```python
from build123d import *
from build123d.topology import SkipClean

# Parameters (mm, degrees)
ESTRUSIONE_ESTRUSIONE1_DEPTH  = 6
ESTRUSIONE_ESTRUSIONE3_START  = -11
SCHIZZO3_R                    = 5
SCHIZZO3_R_2                  = 2.65
ESTRUSIONE_ESTRUSIONE3_DEPTH  = 11
SCHIZZO5_R                    = 0.925
ESTRUSIONE_ESTRUSIONE4_DEPTH  = 20
SCHIZZO12_W                   = 8
SCHIZZO12_H                   = 6
ESTRUSIONE_ESTRUSIONE6_DEPTH  = 2
SCHIZZO13_W                   = 6
SCHIZZO13_H                   = 2
ESTRUSIONE_ESTRUSIONE7_DEPTH  = 3
RACCORDO2_R                   = 2.5
SCHIZZO14_R                   = 1.75
SCHIZZO14_R_2                 = 0.925
TAGLIO_ESTRUSIONE7_DEPTH      = 25
SCHIZZO15_W                   = 6
SCHIZZO15_H                   = 8
ESTRUSIONE_ESTRUSIONE8_DEPTH  = 24
SCHIZZO16_W                   = 6
SCHIZZO16_H                   = 2
ESTRUSIONE_ESTRUSIONE9_DEPTH  = 7.999994
SCHIZZO17_R                   = 1.25
TAGLIO_ESTRUSIONE8_DEPTH      = 25
RACCORDO3_R                   = 10
RACCORDO4_R                   = 10
RACCORDO5_R                   = 10
RACCORDO6_R                   = 2.5
SCHIZZO18_R                   = 1.75
TAGLIO_ESTRUSIONE9_DEPTH      = 39.431359843
SCHIZZO20_W                   = 20
SCHIZZO20_H                   = 19.30891557
TAGLIO_ESTRUSIONE10_DEPTH     = 39.431359843
SCHIZZO21_W                   = 5
SCHIZZO21_H                   = 10
ESTRUSIONE_ESTRUSIONE10_DEPTH = 9.5
SCHIZZO22_W                   = 5
SCHIZZO22_H                   = 10
ESTRUSIONE_ESTRUSIONE11_DEPTH = 15
RACCORDO7_R                   = 5
RACCORDO8_R                   = 10
RACCORDO9_R                   = 5
ESTRUSIONE_ESTRUSIONE13_START = 5
SCHIZZO24_R                   = 5
SCHIZZO24_R_2                 = 2.6
ESTRUSIONE_ESTRUSIONE13_DEPTH = 5
SCHIZZO26_R                   = 1.75
TAGLIO_ESTRUSIONE12_DEPTH     = 39.29124471
RACCORDO10_R                  = 5


with BuildPart() as part:
    # Schizzo1 → Estrusione-Estrusione1 (new body)
    with BuildSketch(Plane.XY):
        with BuildLine():
            Line((0, 0), (-20, 0))
            Line((-20, 0), (-10, 10))
            Line((-10, 10), (10, 10))
            ThreePointArc((10, 10), (15, 5), (10, 0))
            Line((10, 0), (0, 0))
        make_face()
    extrude(amount=ESTRUSIONE_ESTRUSIONE1_DEPTH)

    # Schizzo3 → Estrusione-Estrusione3 (add)
    with SkipClean():  # the faces are left unmerged after this step: merging them gives an invalid solid
        with BuildSketch(Plane.XY.offset(6).offset(ESTRUSIONE_ESTRUSIONE3_START)):
            with Locations(Location((10, 5, 0), (0, 0, 270))):
                Circle(SCHIZZO3_R)
            with Locations((10, 5)):
                Circle(SCHIZZO3_R_2, mode=Mode.SUBTRACT)
        extrude(amount=ESTRUSIONE_ESTRUSIONE3_DEPTH)



with BuildPart() as body_2:
    # Schizzo5 → Estrusione-Estrusione4 (new body)
    with BuildSketch(Plane(origin=(0, 0, 0), x_dir=(-0.7071067811865476, 0.7071067811865476, 0), z_dir=(0.7071067811865476, 0.7071067811865476, 0))):
        with Locations((18.142135624, 3)):
            Circle(SCHIZZO5_R)
    extrude(amount=-ESTRUSIONE_ESTRUSIONE4_DEPTH)

    # Schizzo12 → Estrusione-Estrusione6 (add)
    with BuildSketch(Plane(origin=(0, 0, 0), x_dir=(-0.7071067811865476, 0.7071067811865476, 0), z_dir=(0.7071067811865476, 0.7071067811865476, 0))):
        with Locations((18.142135624, 3)):
            Rectangle(SCHIZZO12_W, SCHIZZO12_H)
    extrude(amount=ESTRUSIONE_ESTRUSIONE6_DEPTH)


with BuildPart() as part_1:
    with SkipClean():  # the faces are left unmerged after this step: merging them gives an invalid solid
        add(part.part)

        add(body_2.part)  # Estrusione-Estrusione7 merges body 2
        # Schizzo13 → Estrusione-Estrusione7 (add)
        with BuildSketch(Plane(origin=(-10, 10, 0), x_dir=(0, 0, -1), z_dir=(0.7071067811865477, -0.7071067811865475, 0))):
            with Locations((-3, 1)):
                Rectangle(SCHIZZO13_W, SCHIZZO13_H)
        extrude(amount=ESTRUSIONE_ESTRUSIONE7_DEPTH)

    # Raccordo2
    raccordo2_edges = [part_1.edges().sort_by_distance(p)[0] for p in [
        (-14.949747468, 16.363961031, 0),
        (-14.949747468, 16.363961031, 6),
    ]]
    fillet(raccordo2_edges, radius=RACCORDO2_R)

    # Schizzo14 → Taglio-Estrusione7 (cut)
    # profile 1 of 2: a face of its own
    with SkipClean():  # the faces are left unmerged after this step: merging them gives an invalid solid
        with BuildSketch(Plane(origin=(1.414213562, 1.414213562, 0), x_dir=(0, 0, -1), z_dir=(0.7071067811865476, 0.7071067811865476, 0))):
            with Locations(Location((-3, 18.142135624, 0), (0, 0, 90))):
                Circle(SCHIZZO14_R)
            with Locations((-3, 18.142135624)):
                Circle(SCHIZZO14_R_2, mode=Mode.SUBTRACT)
        # profile 2 of 2: a face of its own
        with BuildSketch(Plane(origin=(1.414213562, 1.414213562, 0), x_dir=(0, 0, -1), z_dir=(0.7071067811865476, 0.7071067811865476, 0))):
            with Locations((-3, 18.142135624)):
                Circle(SCHIZZO14_R_2)
        extrude(amount=-TAGLIO_ESTRUSIONE7_DEPTH, mode=Mode.SUBTRACT)

    # Schizzo15 → Estrusione-Estrusione8 (add)
    with SkipClean():  # the faces are left unmerged after this step: merging them gives an invalid solid
        with BuildSketch(Plane(origin=(0, 0, 0), x_dir=(0, 0, 1), z_dir=(-0.7071067811865477, -0.7071067811865475, 0))):
            with Locations((3, 10.142135624)):
                Rectangle(SCHIZZO15_W, SCHIZZO15_H)
        extrude(amount=ESTRUSIONE_ESTRUSIONE8_DEPTH)

    # Schizzo16 → Estrusione-Estrusione9 (add)
    with SkipClean():  # the faces are left unmerged after this step: merging them gives an invalid solid
        with BuildSketch(Plane(origin=(-10, 10, 0), x_dir=(0, 0, 1), z_dir=(-0.7071067811865477, 0.7071067811865475, 0))):
            with Locations((3, -23)):
                Rectangle(SCHIZZO16_W, SCHIZZO16_H)
        extrude(amount=ESTRUSIONE_ESTRUSIONE9_DEPTH)

    # Schizzo17 → Taglio-Estrusione8 (cut)
    with SkipClean():  # the faces are left unmerged after this step: merging them gives an invalid solid
        with BuildSketch(Plane(origin=(-16.970562748, -16.970562748, 0), x_dir=(0, 0, 1), z_dir=(-0.7071067811865477, -0.7071067811865474, 0))):
            with Locations(Location((3, 18.142135624, 0), (0, 0, 270))):
                Circle(SCHIZZO17_R)
        extrude(amount=-TAGLIO_ESTRUSIONE8_DEPTH, mode=Mode.SUBTRACT)

    # Raccordo3
    # the kernel refuses this fillet: 10 mm, written as the material it takes off along each edge
    with BuildSketch(Plane(origin=(-21.313708499, -12.627416998, -25), x_dir=(0.7071067811865475, 0.7071067811865475, 0), z_dir=(0, 0, 1))) as raccordo3_piece_1:
        with BuildLine():
            CenterArc((RACCORDO3_R, RACCORDO3_R), RACCORDO3_R, 180, 90)
            Line((0, RACCORDO3_R), (0, 0))
            Line((0, 0), (RACCORDO3_R, 0))
        make_face()
    extrude(amount=56, mode=Mode.SUBTRACT)

    # Raccordo4
    raccordo4_edges = [part_1.edges().sort_by_distance(p)[0] for p in [
        (-8.686291501, 0, 3),
    ]]
    fillet(raccordo4_edges, radius=RACCORDO4_R)

    # Raccordo5
    raccordo5_edges = [part_1.edges().sort_by_distance(p)[0] for p in [
        (-7.171572875, 10, 3),
    ]]
    fillet(raccordo5_edges, radius=RACCORDO5_R)

    # Raccordo6
    raccordo6_edges = [part_1.edges().sort_by_distance(p)[0] for p in [
        (-31.920305974, -0.60660596, 6),
        (-31.920305974, -0.60660596, 0),
    ]]
    fillet(raccordo6_edges, radius=RACCORDO6_R)

    # Schizzo18 → Taglio-Estrusione9 (cut, through all)
    with BuildSketch(Plane.XY.offset(6)):
        with Locations((10, 5)):
            Circle(SCHIZZO18_R)
    extrude(amount=-TAGLIO_ESTRUSIONE9_DEPTH, mode=Mode.SUBTRACT)

    # Schizzo20 → Taglio-Estrusione10 (cut, through all)
    with BuildSketch(Plane(origin=(0, 0, -5), x_dir=(-1, 0, 0), z_dir=(0, 0, -1))):
        with Locations((-10, 5)):
            Rectangle(SCHIZZO20_W, SCHIZZO20_H)
    extrude(amount=-TAGLIO_ESTRUSIONE10_DEPTH, mode=Mode.SUBTRACT)

    # Schizzo21 → Estrusione-Estrusione10 (add)
    with BuildSketch(Plane.XY.offset(6)):
        with Locations((-0.529437252, 5)):
            Rectangle(SCHIZZO21_W, SCHIZZO21_H)
    extrude(amount=ESTRUSIONE_ESTRUSIONE10_DEPTH)

    # Schizzo22 → Estrusione-Estrusione11 (add)
    with BuildSketch(Plane(origin=(1.970562748, 0, 0), x_dir=(0, 0, -1), z_dir=(1, 0, 0))):
        with Locations((-13, 5)):
            Rectangle(SCHIZZO22_W, SCHIZZO22_H)
    extrude(amount=ESTRUSIONE_ESTRUSIONE11_DEPTH)

    # Raccordo7
    # the kernel refuses this fillet: 5 mm, written as the material it takes off along each edge
    with BuildSketch(Plane(origin=(1.970562748, 19.944379675, 6), x_dir=(-1, 0, 0), z_dir=(0, -1, 0))) as raccordo7_piece_1:
        with BuildLine():
            CenterArc((5, -3.97775187), RACCORDO7_R, 127.292729202, 52.707270798)
            Line((0, -3.97775187), (-0.1, -3.97775187))
            Line((-0.1, -3.97775187), (-0.1, 0))
            Line((-0.1, 0), (0, 0.1))
            ThreePointArc((0, 0.1), (0.985281374, 0.1), (1.909974003, 0.079555037))
            Line((1.909974003, 0.079555037), (1.970562748, 0))
        make_face()
    extrude(amount=29.88875935, mode=Mode.SUBTRACT)
    with BuildSketch(Plane(origin=(16.970562748, 0, -2), x_dir=(0, 1, 0), z_dir=(0, 0, 1))) as raccordo7_piece_2:
        with BuildLine():
            CenterArc((RACCORDO7_R, RACCORDO7_R), RACCORDO7_R, 180, 90)
            Line((0, RACCORDO7_R), (-RACCORDO7_R * 0.02, RACCORDO7_R))
            Line((-RACCORDO7_R * 0.02, RACCORDO7_R), (-RACCORDO7_R * 0.02, -RACCORDO7_R * 0.02))
            Line((-RACCORDO7_R * 0.02, -RACCORDO7_R * 0.02), (RACCORDO7_R, -RACCORDO7_R * 0.02))
            Line((RACCORDO7_R, -RACCORDO7_R * 0.02), (RACCORDO7_R, 0))
        make_face()
    extrude(amount=30, mode=Mode.SUBTRACT)
    with BuildSketch(Plane(origin=(16.970562748, 10, 28), x_dir=(-1, 0, 0), z_dir=(0, 0, -1))) as raccordo7_piece_3:
        with BuildLine():
            CenterArc((RACCORDO7_R, -RACCORDO7_R), RACCORDO7_R, 90, 90)
            Line((0, -RACCORDO7_R), (-RACCORDO7_R * 0.02, -RACCORDO7_R))
            Line((-RACCORDO7_R * 0.02, -RACCORDO7_R), (-RACCORDO7_R * 0.02, RACCORDO7_R * 0.02))
            Line((-RACCORDO7_R * 0.02, RACCORDO7_R * 0.02), (RACCORDO7_R, RACCORDO7_R * 0.02))
            Line((RACCORDO7_R, RACCORDO7_R * 0.02), (RACCORDO7_R, 0))
        make_face()
    extrude(amount=30, mode=Mode.SUBTRACT)

    # Raccordo8
    # the kernel refuses this fillet: 10 mm, written as the material it takes off along each edge
    with BuildSketch(Plane(origin=(-3.029437252, -24.968730444, 15.5), x_dir=(1, 0, 0), z_dir=(0, 1, 0))) as raccordo8_piece_1:
        with BuildLine():
            CenterArc((9.987492178, 10), RACCORDO8_R, 182.865983983, 87.134016017)
            Line((0, 9.5), (-0.199749844, 9.49))
            ThreePointArc((-0.199749844, 9.49), (-0.2, 4.75), (-0.2, 0))
            Line((-0.2, 0), (0, -0.2))
            Line((0, -0.2), (9.987492178, -0.2))
            Line((9.987492178, -0.2), (9.987492178, 0))
        make_face()
    extrude(amount=59.937460889, mode=Mode.SUBTRACT)

    # Raccordo9
    raccordo9_edges = [part_1.edges().sort_by_distance(p)[0] for p in [
        (-3.029437252, 5, 6),
    ]]
    fillet(raccordo9_edges, radius=RACCORDO9_R)

    # Schizzo24 → Estrusione-Estrusione13 (add)
    with BuildSketch(Plane(origin=(0, 0, 10.5), x_dir=(-1, 0, 0), z_dir=(0, 0, -1)).offset(ESTRUSIONE_ESTRUSIONE13_START)):
        with Locations(Location((-11.970562748, 5, 0), (0, 0, 180))):
            Circle(SCHIZZO24_R)
        with Locations((-11.970562748, 5)):
            Circle(SCHIZZO24_R_2, mode=Mode.SUBTRACT)
    extrude(amount=-ESTRUSIONE_ESTRUSIONE13_DEPTH)

    # Schizzo26 → Taglio-Estrusione12 (cut, through all)
    with BuildSketch(Plane(origin=(0, 0, 10.5), x_dir=(-1, 0, 0), z_dir=(0, 0, -1))):
        with Locations((-11.970562748, 5)):
            Circle(SCHIZZO26_R)
    extrude(amount=-TAGLIO_ESTRUSIONE12_DEPTH, mode=Mode.SUBTRACT)

    # Raccordo10
    raccordo10_edges = [part_1.edges().sort_by_distance(p)[0] for p in [
        (0, 5, 6),
        (1.970562748, 5, 10.5),
    ]]
    fillet(raccordo10_edges, radius=RACCORDO10_R)


solid = part_1.part
```
Read the model definition and answer for the solid it produces. Units are mm, in the model's axes. A direction names the side the tool comes from. Round coordinates to 2 decimals unless told otherwise and drop trailing zeros. Write each loop counter-clockwise with the first axis right and the second up, starting at its lowest first coordinate (ties: lowest second). Pieces come first, ordered by that corner, then holes. Notation, with made-up numbers: (12.5, -31.75) - (43.5, -31.75) arc R20 ccw to (43.5, 3.25) - close; hole circle Ø7 at (-4, 37). An arc over 180 degrees is marked (long way). One line per item, written item: value.
Q1. For a pull along X with two mould halves and no side action, classify faces 4 (the cylindrical face through (-4, 5, 7)), 5 (the flat face through (0, 5, 2)), 6 (the cylindrical face through (9.49, 5.78, 7.96)) as pulls with the +X half, pulls with the -X half, needs draft (parallel to the pull), parting line crosses it, or undercut.
The answers:
face 4: pulls with the -X half
face 5: pulls with the +X half
face 6: undercut
Q2. Which of the six approach directions +Z, -Z, +X, -X, +Y, -Y give full straight-line access (tool end or side, diameter ignored) to faces 1 (the flat face through (6.5, 5, 10.5)), 2 (the flat face through (2, 0, 10)), 3 (the flat face through (-16, 1, 6))?
The answers:
face 1: -Z
face 2: +Z, -Z, +X, -Y
face 3: +Z, -X, +Y, -Y
Q3. Find section B-B (x = -27). Determine the outline of the cut face in (y, z), and give its area (3 significant figures).
The answers:
outline: (-6.71, 0) - (-4.11, 0) - (-4.11, 6) - (-6.71, 6) - close
area: 15.6 mm2
Q4. Find section A-A (z = 11.5). Determine the outline of the cut face in (x, y).
The answers:
outline: (-1.04, 0) - (11.97, 0) arc R5 ccw to (11.97, 10) - (-1.04, 10) - close; hole circle Ø3.5 at (11.97, 5)
Q5. Straight lines are drawn through the part: line 1 (Y direction, x = -0.5, z = 6); line 2 (Z direction, x = -1.5, y = 2); line 3 (X direction, y = 5.25, z = 8.5). For each, find the intervals that lie inside material, in ascending order. Write a range as from..to.
The answers:
line 1: y = 0..10
line 2: z = 0..10.83
line 3: x = -2.67..1.91, 6.98..9.38, 14.56..16.96
Q6. Each of these flat-tipped pins is pushed along its axis until it touches: P1, Ø4.5, axis at x = 11.97, y = 5, coming from the -Z side; P2, Ø4, axis at x = -22, y = 3, coming from the +Z side; P3, Ø12, axis at x = -16.5, y = 0.5, coming from the +Z side; P4, Ø1.2, axis at y = 4.5, z = 2, coming from the +X side. Where does it stop, or does it pass through?
The answers:
P1: stops at z = 10.5
P2: passes through
P3: stops at z = 6
P4: stops at x = 0
